```python
from build123d import *

# Parameters (mm, degrees)
EXTRUDE_4_DEPTH = 40


with BuildPart() as part:
    # 草图2 → 凸台-拉伸4 (new body)
    with BuildSketch(Plane.XY):
        with BuildLine():
            Line((55.601230388, 2.559909891), (273.486476264, 2.559909891))
            Line((273.486476264, 2.559909891), (273.486476264, -2.559909891))
            Line((273.486476264, -2.559909891), (55.601230388, -2.559909891))
            ThreePointArc((55.601230388, -2.559909891), (-55.660128991, 0), (55.601230388, 2.559909891))
        make_face()
        with BuildLine():
            ThreePointArc((32.799591871, 2.559909891), (0, 32.899336856), (-32.799591871, 2.559909891))
            Line((-32.799591871, 2.559909891), (-24.758977016, 2.559909891))
            ThreePointArc((-24.758977016, 2.559909891), (0, 24.890963853), (24.758977016, 2.559909891))
            Line((24.758977016, 2.559909891), (32.799591871, 2.559909891))
        make_face(mode=Mode.SUBTRACT)
        with BuildLine():
            Line((-48.158715074, -2.559909891), (-40.845588283, -2.559909891))
            ThreePointArc((-40.845588283, -2.559909891), (0, -40.925728104), (40.845588283, -2.559909891))
            Line((40.845588283, -2.559909891), (48.158715074, -2.559909891))
            ThreePointArc((48.158715074, -2.559909891), (0, -48.226703974), (-48.158715074, -2.559909891))
        make_face(mode=Mode.SUBTRACT)
        with BuildLine():
            Line((40.845588283, 2.559909891), (48.158715074, 2.559909891))
            ThreePointArc((48.158715074, 2.559909891), (0, 48.226703974), (-48.158715074, 2.559909891))
            Line((-48.158715074, 2.559909891), (-40.845588283, 2.559909891))
            ThreePointArc((-40.845588283, 2.559909891), (0, 40.925728104), (40.845588283, 2.559909891))
        make_face(mode=Mode.SUBTRACT)
        with BuildLine():
            Line((-32.799591871, -2.559909891), (-24.758977016, -2.559909891))
            ThreePointArc((-24.758977016, -2.559909891), (0, -24.890963853), (24.758977016, -2.559909891))
            Line((24.758977016, -2.559909891), (32.799591871, -2.559909891))
            ThreePointArc((32.799591871, -2.559909891), (0, -32.899336856), (-32.799591871, -2.559909891))
        make_face(mode=Mode.SUBTRACT)
    extrude(amount=EXTRUDE_4_DEPTH)


solid = part.part
```
Can you work these out from the model? Positions are in its coordinate system, mm. A direction names the side the tool comes from. Coordinates: 2 decimals unless noted, no trailing zeros. Loops run counter-clockwise (first coordinate to the right, second up) from the corner with the lowest first, then second, coordinate; pieces in that order, holes last. Notation, with made-up numbers: (-4, 59.5) - (51, 59.5) arc R31 ccw to (51, 87.5) - close; hole circle Ø7 at (-2.75, 51.25). An arc over 180 degrees is marked (long way). Use a Markdown table: item, result.
Item 1: If I drill on probe 1 along Y at (x, z) = (-22.5, 3.5); probe 2 along X at (y, z) = (10, 6); probe 3 along X at (y, z) = (34.5, 15), over which ranges is the centre line in solid material (lowest first)? Write a range as from..to.
Numbers:
| item | result |
|---|---|
| probe 1 | y = -50.91..-42.66, -34.19..-24, -10.64..10.64, 24..34.19, 42.66..50.91 |
| probe 2 | x = -54.75..-47.18, -39.69..-31.34, -22.79..22.79, 31.34..39.69, 47.18..54.75 |
| probe 3 | x = -43.68..-33.7, -22.02..22.02, 33.7..43.68 |
Item 2: Will these pins go through, and if not, where does the flat tip stop? pin 1 (6 mm diameter, centred on x = -44, z = 11.5, fed in from +Y); pin 2 (6.5 mm diameter, centred on x = 27.5, z = 25.5, fed in from +Y); pin 3 (8 mm diameter, centred on x = -46, z = 21, fed in from -Y); pin 4 (6 mm diameter, centred on x = 59.5, y = 10.5, fed in from +Z).
Numbers:
| item | result |
|---|---|
| pin 1 | stops at y = 37.64 |
| pin 2 | stops at y = 50.1 |
| pin 3 | stops at y = -36.52 |
| pin 4 | passes through |
Item 3: I want a section at C-C on z = 4.5. Please give me the cut outline in (x, y).
Numbers:
| item | result |
|---|---|
| outline | (55.6, -2.56) - (273.49, -2.56) - (273.49, 2.56) - (55.6, 2.56) arc R55.66 ccw (long way) to start; hole (-48.16, -2.56) arc R48.23 ccw to (48.16, -2.56) - (40.85, -2.56) arc R40.93 cw to (-40.85, -2.56) - close; hole (-48.16, 2.56) - (-40.85, 2.56) arc R40.93 cw to (40.85, 2.56) - (48.16, 2.56) arc R48.23 ccw to start; hole (-32.8, -2.56) arc R32.9 ccw to (32.8, -2.56) - (24.76, -2.56) arc R24.89 cw to (-24.76, -2.56) - close; hole (-32.8, 2.56) - (-24.76, 2.56) arc R24.89 cw to (24.76, 2.56) - (32.8, 2.56) arc R32.9 ccw to start |
Item 4: I want a section at A-A on x = 0. Please give me the cut outline in (y, z), and give its area (3 significant figures).
Numbers:
| item | result |
|---|---|
| outline | (-55.66, 0) - (-48.23, 0) - (-48.23, 40) - (-55.66, 40) - close; (-40.93, 0) - (-32.9, 0) - (-32.9, 40) - (-40.93, 40) - close; (-24.89, 0) - (24.89, 0) - (24.89, 40) - (-24.89, 40) - close; (32.9, 0) - (40.93, 0) - (40.93, 40) - (32.9, 40) - close; (48.23, 0) - (55.66, 0) - (55.66, 40) - (48.23, 40) - close |
| area | 3,230 mm2 |
Item 5: I want a section at B-B on y = -14. Please give me the cut outline in (x, z).
Numbers:
| item | result |
|---|---|
| outline | (-53.87, 0) - (-46.15, 0) - (-46.15, 40) - (-53.87, 40) - close; (-38.46, 0) - (-29.77, 0) - (-29.77, 40) - (-38.46, 40) - close; (-20.58, 0) - (20.58, 0) - (20.58, 40) - (-20.58, 40) - close; (29.77, 0) - (38.46, 0) - (38.46, 40) - (29.77, 40) - close; (46.15, 0) - (53.87, 0) - (53.87, 40) - (46.15, 40) - close |
Item 6: For faces 4 (the face through (1.025, -48.216, 19.72)), 5 (the face through (163, 2.56, 20)), which set-ups out of +Z, -Z, +X, -X, +Y, -Y let a thin tool reach every point of the face, with its end or its side?
Numbers:
| item | result |
|---|---|
| face 4 | +Z, -Z |
| face 5 | +Z, -Z, +X, +Y |
Item 7: I want a section at D-D on y = 37. Please give me the cut outline in (x, z).
Numbers:
| item | result |
|---|---|
| outline | (-41.58, 0) - (-30.93, 0) - (-30.93, 40) - (-41.58, 40) - close; (-17.49, 0) - (17.49, 0) - (17.49, 40) - (-17.49, 40) - close; (30.93, 0) - (41.58, 0) - (41.58, 40) - (30.93, 40) - close |
Item 8: We'd pull the mould along X, two halves only. Please class faces 1 (the face through (-55.608, -2.411, 19.72)), 2 (the face through (24, -4, 0)), 3 (the face through (-29, -2.56, 20)): released by +X, released by -X, zero draft, split by the parting line, or undercut.
Numbers:
| item | result |
|---|---|
| face 1 | split by the parting line |
| face 2 | zero draft |
| face 3 | undercut |
